Work out the finished part from the listing and answer in its coordinate system (mm). A direction names the side the tool comes from. Coordinates: 2 decimals unless noted, no trailing zeros. Order: outer loops, then holes, each group sorted by start corner. A loop starts at its lowest first (then second) coordinate and runs counter-clockwise, first axis right, second up. Notation, with made-up numbers: (7.5, 11.25) -> (18.5, 11.25) arc R33 cw to (18.5, 44.25) -> close; hole circle Ø3 at (-38.5, -8.75). An arc over 180 degrees is marked (long way). Answer as CSV lines item,"result". Start each with the question number.
Item 1: Section C-C (x = 11.75) is taken. Write down the section's boundary in (y, z), then the cut area to 3 significant figures.
Item 2: Section A-A (z = -14) is taken. Write down the section's boundary in (x, y).
Item 3: Which of the six approach directions +Z, -Z, +X, -X, +Y, -Y give full straight-line access (tool end or side, diameter ignored) to faces 4 (the face through (-1, 6, -31)), 5 (the face through (-0.5, 10.4, -26.9)), 6 (the face through (10, 3.04, -10)), 7 (the face through (1, 5.04, -17)), 8 (the face through (2.96, 2.56, -21.38))?
Item 4: For a pull along Z with two mould halves and no side action, classify faces 1 (the face through (3.53, 2.56, -3.35)), 2 (the face through (10, 23, -28)), 3 (the face through (20.5, 10.7, -35.831)) as pulls with the +Z half, pulls with the -Z half, needs draft (parallel to the pull), parting line crosses it, or undercut.
Item 5: Each of these flat-tipped pins is pushed along its axis until it touches: pin 1 Ø2 at (x, z) = (16.39, -22.95) entering from -Y; pin 2 Ø4 at (x, z) = (3.5, -23) entering from +Y; pin 3 Ø4.5 at (y, z) = (2.5, -11.5) entering from -X; pin 4 Ø8 at (y, z) = (24.5, -30.5) entering from +X. Where does it stop, or does it pass through?
Item 6: Straight lines are drawn through the part: L1, parallel to Y at x = 15.5, z = -29.75; L2, parallel to X at y = 3.7, z = -14; L3, parallel to Y at x = 15, z = -31.5. For each, find the intervals that lie inside material, in ascending order.
Item 7: Section B-B (y = 35.54) is taken. Write down the section's boundary in (x, z), then the cut area to 3 significant figures.
Item 8: Section D-D (x = 4.5) is taken. Count the separate pieces of the cut face and the enclosed holes in it, then the cut area to 3 significant figures.
```python
from build123d import *

# Parameters (mm, degrees)
SKETCH1_W           = 20
SKETCH1_H           = 28
BOSS_EXTRUDE1_DEPTH = 5.04
SKETCH3_R           = 9
CUT_EXTRUDE1_DEPTH  = 2
SKETCH4_R           = 3
CUT_EXTRUDE2_DEPTH  = 35.543329313
SKETCH7_R           = 1.7
CUT_EXTRUDE3_DEPTH  = 35.776451803
BOSS_EXTRUDE2_DEPTH = 8.331
SKETCH9_R           = 1.7
CUT_EXTRUDE4_DEPTH  = 54.556340428
FILLET2_R           = 0.5
BOSS_EXTRUDE3_DEPTH = 1
BOSS_EXTRUDE4_DEPTH = 1


with BuildPart() as part:
    # Sketch1 → Boss-Extrude1 (new body)
    with BuildSketch(Plane(origin=(0, 0, 0), x_dir=(1, 0, 0), z_dir=(0, 1, 0))):
        with Locations((10, 14)):
            Rectangle(SKETCH1_W, SKETCH1_H)
    extrude(amount=BOSS_EXTRUDE1_DEPTH)

    # Sketch3 → Cut-Extrude1 (cut)
    with BuildSketch(Plane(origin=(0, 5.04, 0), x_dir=(1, 0, 0), z_dir=(0, 1, 0))):
        with Locations(Location((10, 14, 0), (0, 0, 270))):
            Circle(SKETCH3_R)
    extrude(amount=-CUT_EXTRUDE1_DEPTH, mode=Mode.SUBTRACT)

    # Sketch4 → Cut-Extrude2 (cut, through all)
    with BuildSketch(Plane(origin=(0, 3.04, 0), x_dir=(1, 0, 0), z_dir=(0, 1, 0))):
        with Locations(Location((10, 14, 0), (0, 0, 270))):
            Circle(SKETCH4_R)
    extrude(amount=-CUT_EXTRUDE2_DEPTH, mode=Mode.SUBTRACT)

    # Sketch7 → Cut-Extrude3 (cut, through all)
    with BuildSketch(Plane(origin=(0, 5.04, 0), x_dir=(1, 0, 0), z_dir=(0, 1, 0))):
        with Locations(Location((3.607579394, 22.951924866, 0), (0, 0, 270))):
            Circle(SKETCH7_R)
        with Locations(Location((16.392420606, 22.951924866, 0), (0, 0, 90))):
            Circle(SKETCH7_R)
        with Locations(Location((16.392420606, 5.048075134, 0), (0, 0, 270))):
            Circle(SKETCH7_R)
        with Locations(Location((3.607579394, 5.048075134, 0), (0, 0, 90))):
            Circle(SKETCH7_R)
    extrude(amount=-CUT_EXTRUDE3_DEPTH, mode=Mode.SUBTRACT)

    # Sketch8 → Boss-Extrude2 (add)
    with BuildSketch(Plane(origin=(0, 0, -28), x_dir=(-1, 0, 0), z_dir=(0, 0, -1))):
        Polygon((-20, 5.04), (-20, 41.04), (0, 41.04), (0, 5.04), (0, 0), (-20, 0), align=None)
    extrude(amount=BOSS_EXTRUDE2_DEPTH)

    # Sketch9 → Cut-Extrude4 (cut, through all)
    with BuildSketch(Plane.XY.offset(-28)):
        with Locations((4.5, 10.54)):
            Circle(SKETCH9_R)
        with Locations(Location((15.5, 10.54, 0), (0, 0, 180))):
            Circle(SKETCH9_R)
        with Locations((15.5, 35.54)):
            Circle(SKETCH9_R)
        with Locations(Location((4.5, 35.54, 0), (0, 0, 180))):
            Circle(SKETCH9_R)
    extrude(amount=-CUT_EXTRUDE4_DEPTH, mode=Mode.SUBTRACT)

    # Fillet2
    fillet2_edges = [part.edges().sort_by_distance(p)[0] for p in [
        (20, 5.04, -14),
        (10, 5.04, -28),
        (0, 23.04, -28),
        (10, 41.04, -28),
        (0, 41.04, -32.1655),
        (20, 23.04, -28),
        (20, 41.04, -32.1655),
        (20, 20.52, -36.331),
        (10, 0, -36.331),
        (0, 20.52, -36.331),
        (10, 41.04, -36.331),
        (0, 5.04, -14),
        (20, 0, -18.1655),
        (10, 0, 0),
        (0, 0, -18.1655),
        (20, 2.52, 0),
        (0, 2.52, 0),
        (10, 5.04, 0),
    ]]
    fillet(fillet2_edges, radius=FILLET2_R)

    # Sketch10 → Boss-Extrude3 (add)
    with BuildSketch(Plane(origin=(20, 0, 0), x_dir=(0, 0, -1), z_dir=(1, 0, 0))):
        Polygon((18.1655, 0.5), (35.831, 20.52), (35.831, 0.5), align=None)
    extrude(amount=BOSS_EXTRUDE3_DEPTH)

    # Sketch11 → Boss-Extrude4 (add)
    with BuildSketch(Plane.ZY):
        Polygon((-18.1655, 0.5), (-35.831, 20.52), (-35.831, 0.5), align=None)
    extrude(amount=BOSS_EXTRUDE4_DEPTH)


solid = part.part
```
Checked values:
1,outline,"(0, -35.83) arc R0.5 ccw to (0.5, -36.33) -> (40.54, -36.33) arc R0.5 ccw to (41.04, -35.83) -> (41.04, -28.5) arc R0.5 ccw to (40.54, -28) -> (5.54, -28) arc R0.5 cw to (5.04, -27.5) -> (5.04, -22.83) -> (3.04, -22.83) -> (3.04, -16.44) -> (0, -16.44) -> close; (0, -11.56) -> (3.04, -11.56) -> (3.04, -5.17) -> (5.04, -5.17) -> (5.04, -0.5) arc R0.5 ccw to (4.54, 0) -> (0.5, 0) arc R0.5 ccw to (0, -0.5) -> close"
1,area,"433 mm^2"
2,outline,"(0, 0.5) arc R0.5 ccw to (0.5, 0) -> (7, 0) -> (7, 3.04) -> (1, 3.04) -> (1, 5.04) -> (0.5, 5.04) arc R0.5 ccw to (0, 4.54) -> close; (13, 0) -> (19.5, 0) arc R0.5 ccw to (20, 0.5) -> (20, 4.54) arc R0.5 ccw to (19.5, 5.04) -> (19, 5.04) -> (19, 3.04) -> (13, 3.04) -> close"
3,face 4,"+Z, -Z, -X, +Y, -Y"
3,face 5,"+Z, -X, +Y"
3,face 6,"+Y"
3,face 7,"+Z, +Y"
3,face 8,"+Y, -Y"
4,face 1,"undercut"
4,face 2,"pulls with the +Z half"
4,face 3,"pulls with the -Z half"
5,pin 1,"passes through"
5,pin 2,"stops at y = 5.04"
5,pin 3,"stops at x = 0"
5,pin 4,"stops at x = 20"
6,L1,"y = 0 to 8.84, 12.24 to 33.84, 37.24 to 41.04"
6,L2,"x = 0 to 1, 19 to 20"
6,L3,"y = 0 to 8.92, 12.16 to 33.92, 37.16 to 41.04"
7,outline,"(0, -35.83) arc R0.5 ccw to (0.5, -36.33) -> (2.8, -36.33) -> (2.8, -28) -> (0.5, -28) arc R0.5 ccw to (0, -28.5) -> close; (6.2, -36.33) -> (13.8, -36.33) -> (13.8, -28) -> (6.2, -28) -> close; (17.2, -36.33) -> (19.5, -36.33) arc R0.5 ccw to (20, -35.83) -> (20, -28.5) arc R0.5 ccw to (19.5, -28) -> (17.2, -28) -> close"
7,area,"110 mm^2"
8,separate pieces,"5"
8,enclosed holes,"0"
8,area,"368 mm^2"
